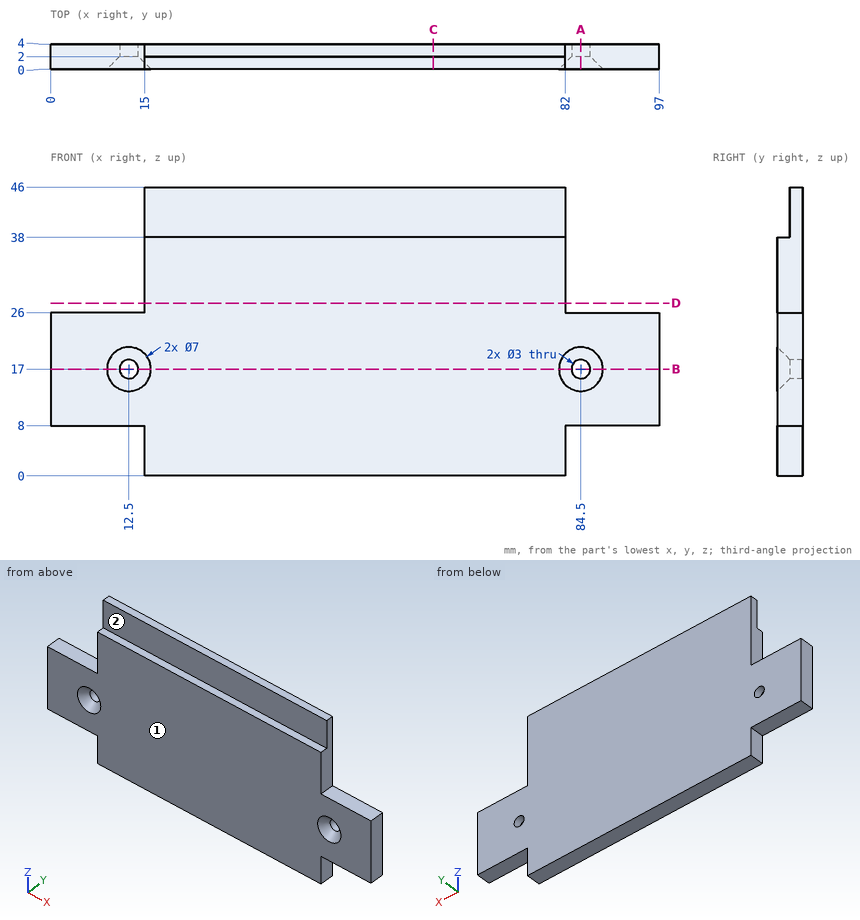
The drawing under review shows one solid part. Ordinate dimensions are in mm from its lowest x, y, z. A direction names the side the tool comes from. Give positions to 0.01 mm unless a question says otherwise; leave off trailing zeros. Write each loop counter-clockwise with the first axis right and the second up, starting at its lowest first coordinate (ties: lowest second). Pieces come first, ordered by that corner, then holes. Notation, with made-up numbers: (69, 71) -> (89, 71) arc R26 cw to (89, 86) -> close; hole circle Ø2 at (-40, 39.25). An arc over 180 degrees is marked (long way). Answer in a Markdown table with one row per item.
(1) Consider section A-A (x = 84.5). State the section outline as (y, z) points, then the cut area to 3 significant figures.
Results:
| item | result |
|---|---|
| outline | (0, 8) -> (4, 8) -> (4, 15.5) -> (2, 15.5) -> (0, 13.5) -> close; (0, 20.5) -> (2, 18.5) -> (4, 18.5) -> (4, 26) -> (0, 26) -> close |
| area | 56.0 mm2 |
(2) For the marked faces 1 and 2, list the 3-axis set-ups (+Z, -Z, +X, -X, +Y, -Y) from which the entire face can be reached by the end or side of a thin tool; tool diameter is ignored.
Results:
| item | result |
|---|---|
| face 1 | +Z, -Z, +X, -X, -Y |
| face 2 | +Z, +X, -X, -Y |
(3) Consider section B-B (z = 17). State the section outline as (x, y) points, then the cut area to 3 significant figures.
Results:
| item | result |
|---|---|
| outline | (0, 0) -> (9, 0) -> (11, 2) -> (11, 4) -> (0, 4) -> close; (14, 2) -> (16, 0) -> (81, 0) -> (83, 2) -> (83, 4) -> (14, 4) -> close; (86, 2) -> (88, 0) -> (97, 0) -> (97, 4) -> (86, 4) -> close |
| area | 356 mm2 |
(4) Clearance check with flat-ended pins moving along their axes: pin 1 (2 mm diameter, centred on x = 91, y = 2.5, fed in from +Z); pin 2 (2 mm diameter, centred on x = 64, y = 0.5, fed in from +Z); pin 3 (1.2 mm diameter, centred on y = 1.5, z = 38.5, fed in from -X). State where each tip first meets the part, or that it passes through.
Results:
| item | result |
|---|---|
| pin 1 | z = 26 |
| pin 2 | z = 38 |
| pin 3 | x = 15 |
(5) Consider section C-C (x = 61). State the section outline as (y, z) points, then the cut area to 3 significant figures.
Results:
| item | result |
|---|---|
| outline | (0, 0) -> (4, 0) -> (4, 46) -> (2, 46) -> (2, 38) -> (0, 38) -> close |
| area | 168 mm2 |
(6) Consider section D-D (z = 27.5). State the section outline as (x, y) points.
Results:
| item | result |
|---|---|
| outline | (15, 0) -> (82, 0) -> (82, 4) -> (15, 4) -> close |
(7) To check wall thickness, follow probe 1 along Z at (x, y) = (12.5, 3.4); probe 2 along Z at (x, y) = (9, 2.7); probe 3 along X at (y, z) = (2.8, 39). State the ranges of each line that lie inside material, in increasing order.
Results:
| item | result |
|---|---|
| probe 1 | 8 to 15.5, 18.5 to 26 |
| probe 2 | 8 to 26 |
| probe 3 | 15 to 82 |
